```python
from build123d import *

# Parameters (mm, degrees)
SKETCH_1_W          = 61.5
SKETCH_1_H          = 37.5
SKETCH_1_W_2        = 55.5
SKETCH_1_H_2        = 33
EXTRUDE_2_DEPTH     = 2
SKETCH_1_4_W        = 67.5
SKETCH_1_4_H        = 43.5
SKETCH_1_4_W_2      = 61.5
SKETCH_1_4_H_2      = 37.5
EXTRUDE_3_DEPTH     = 15
SKETCH_1_5_W        = 67.5
SKETCH_1_5_H        = 43.5
EXTRUDE_4_DEPTH     = 3
CUT_EXTRUDE_1_REACH = 5
SKETCH_1_6_W        = 4.5
SKETCH_1_6_H        = 4.5
SKETCH_3_W          = 64.5
SKETCH_3_H          = 40.5
CUT_EXTRUDE_2_DEPTH = 1
SKETCH_4_W          = 20
SKETCH_4_H          = 20
CUT_EXTRUDE_4_DEPTH = 4


with BuildPart() as part:
    # Sketch 1 → Extrude 2 (new body)
    with BuildSketch(Plane(origin=(0, 0, 0), x_dir=(1, 0, 0), z_dir=(0, 1, 0))):
        with Locations((-28.437260101, -18.832094604)):
            Rectangle(SKETCH_1_W, SKETCH_1_H)
        with Locations((-28.437260101, -19.582094604)):
            Rectangle(SKETCH_1_W_2, SKETCH_1_H_2, mode=Mode.SUBTRACT)
    extrude(amount=EXTRUDE_2_DEPTH)

    # Sketch 1_4 → Extrude 3 (add)
    with BuildSketch(Plane(origin=(0, 0, 0), x_dir=(1, 0, 0), z_dir=(0, 1, 0))):
        with Locations((-28.437260101, -18.832094604)):
            Rectangle(SKETCH_1_4_W, SKETCH_1_4_H)
        with Locations((-28.437260101, -18.832094604)):
            Rectangle(SKETCH_1_4_W_2, SKETCH_1_4_H_2, mode=Mode.SUBTRACT)
    extrude(amount=EXTRUDE_3_DEPTH)

    # Sketch 1_5 → Extrude 4 (add)
    with BuildSketch(Plane(origin=(0, 0, 0), x_dir=(1, 0, 0), z_dir=(0, 1, 0))):
        with Locations((-28.437260101, -18.832094604)):
            Rectangle(SKETCH_1_5_W, SKETCH_1_5_H)
    extrude(amount=-EXTRUDE_4_DEPTH)

    # Sketch 1_6 → Cut-Extrude 1 (cut, up to next)
    with BuildSketch(Plane(origin=(0, 0, 0), x_dir=(1, 0, 0), z_dir=(0, 1, 0)), mode=Mode.PRIVATE) as cut_extrude_1_sk1:
        with Locations((-7.437260101, -32.782094604)):
            Rectangle(SKETCH_1_6_W, SKETCH_1_6_H)
    cut_extrude_1_tool1 = extrude(cut_extrude_1_sk1.sketch, amount=-CUT_EXTRUDE_1_REACH, mode=Mode.PRIVATE) & part.part
    add(cut_extrude_1_tool1.solids().sort_by_distance((-7.43726, 0, 32.782095))[0], mode=Mode.SUBTRACT)

    # Sketch 3 → Cut-Extrude 2 (cut)
    with BuildSketch(Plane(origin=(0, 15, 0), x_dir=(1, 0, 0), z_dir=(0, 1, 0))):
        with Locations((-28.437260101, -18.832094604)):
            Rectangle(SKETCH_3_W, SKETCH_3_H)
    extrude(amount=-CUT_EXTRUDE_2_DEPTH, mode=Mode.SUBTRACT)

    # Sketch 4 → Cut-Extrude 4 (cut, through all)
    with BuildSketch(Plane(origin=(0, 0, 0), x_dir=(1, 0, 0), z_dir=(0, 1, 0))):
        with Locations((-26.4581734, -13.054729736)):
            Rectangle(SKETCH_4_W, SKETCH_4_H)
    extrude(amount=-CUT_EXTRUDE_4_DEPTH, mode=Mode.SUBTRACT)


solid = part.part
```
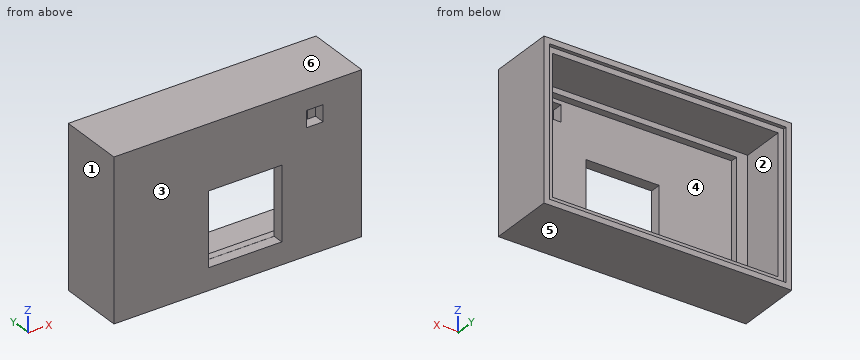
The model under review builds one solid part; all positions refer to its coordinate system, in mm. Face numbers are marked on the shaded views. A direction names the side the tool comes from. Round coordinates to 2 decimals unless told otherwise and drop trailing zeros. Order: outer loops, then holes, each group sorted by start corner. A loop starts at its lowest first (then second) coordinate and runs counter-clockwise, first axis right, second up. Notation, with made-up numbers: (56, -35.75) - (107, -35.75) arc R12 cw to (107, -25.75) - close; hole circle Ø8 at (74.25, 5). An arc over 180 degrees is marked (long way). Answer in a Markdown table with one row per item.
(1) Clearance check with flat-ended pins moving along their axes: P1, Ø11, axis at x = -37.5, z = 16.5, coming from the +Y side; P2, Ø20, axis at x = -16.5, z = 28, coming from the +Y side. State where each tip first meets the part, or that it passes through.
Result set:
| item | result |
|---|---|
| P1 | stops at y = 0 |
| P2 | stops at y = 14 |
(2) Machinability: for the marked faces 1 and 2, which of the approach directions +Z, -Z, +X, -X, +Y, -Y give a long, thin tool a straight path to every point of the face, cutting with its end or side? Answer none if there is none.
Result set:
| item | result |
|---|---|
| face 1 | +Z, -Z, -X, +Y, -Y |
| face 2 | +Y |
(3) For line 1 (Z direction, x = -15.5, y = 7.5); line 2 (X direction, y = -1, z = 7); line 3 (X direction, y = 2.5, z = 2), list the stretches that pass through material, from the lowest coordinate up. Write a range as from..to.
Result set:
| item | result |
|---|---|
| line 1 | z = -2.92..0.08, 37.58..40.58 |
| line 2 | x = -62.19..-36.46, -16.46..5.31 |
| line 3 | x = -62.19..-59.19, 2.31..5.31 |
(4) Mouldability with a two-part tool opening along Z and no side actions: class the marked faces 3, 4, 5 and 6 as released by +Z, released by -Z, zero draft, split by the parting line, or undercut.
Result set:
| item | result |
|---|---|
| face 3 | zero draft |
| face 4 | undercut |
| face 5 | released by -Z |
| face 6 | released by +Z |
(5) Take a section at D-D on x = -40. Write out the cut boundary in (y, z).
Result set:
| item | result |
|---|---|
| outline | (-3, -2.92) - (15, -2.92) - (15, -1.42) - (14, -1.42) - (14, 0.08) - (2, 0.08) - (2, 3.08) - (0, 3.08) - (0, 36.08) - (2, 36.08) - (2, 37.58) - (14, 37.58) - (14, 39.08) - (15, 39.08) - (15, 40.58) - (-3, 40.58) - close |
(6) Take a section at C-C on y = 1. Write out the cut boundary in (x, z), plus the area to 3 significant figures.
Result set:
| item | result |
|---|---|
| outline | (-62.19, -2.92) - (5.31, -2.92) - (5.31, 40.58) - (-62.19, 40.58) - close; hole (-56.19, 3.08) - (-0.69, 3.08) - (-0.69, 36.08) - (-56.19, 36.08) - close |
| area | 1,100 mm2 |
(7) Take a section at A-A on z = 20. Write out the cut boundary in (x, y).
Result set:
| item | result |
|---|---|
| outline | (-62.19, -3) - (-36.46, -3) - (-36.46, 0) - (-56.19, 0) - (-56.19, 2) - (-59.19, 2) - (-59.19, 14) - (-60.69, 14) - (-60.69, 15) - (-62.19, 15) - close; (-16.46, -3) - (5.31, -3) - (5.31, 15) - (3.81, 15) - (3.81, 14) - (2.31, 14) - (2.31, 2) - (-0.69, 2) - (-0.69, 0) - (-16.46, 0) - close |
